from build123d import *

# Parameters (mm, degrees)
F1_DEPTH = 35
F2_DEPTH = 22.5
F5_DEPTH = 2
F7_D     = 2.4
F7_DEPTH = 18
F7_TIP   = 0.7210327428
F10_D    = 5


with BuildPart() as f1:
    # F0 (on Front) → F1 (new body, symmetric)
    with BuildSketch(Plane.XZ):
        with BuildLine():
            ThreePointArc((-74.9516211859, 11.7238655704), (-51.6668855763, 17.075104802), (-41.558504512, -4.5728813857))
            Line((-41.558504512, -4.5728813857), (-28.4346174449, -4.5728813857))
            Line((-28.4346174449, -4.5728813857), (-28.4346174449, -17.4488071352))
            Line((-28.4346174449, -17.4488071352), (-26.8566174449, -19.9622381479))
            Line((-26.8566174449, -19.9622381479), (-13.633294031, -19.9622381479))
            Line((-13.633294031, -19.9622381479), (-12.0557677819, -17.4488071352))
            Line((-12.0557677819, -17.4488071352), (-12.0557677819, -3.6602381479))
            Line((-12.0557677819, -3.6602381479), (8.6728588212, -3.6602381479))
            Line((8.6728588212, -3.6602381479), (8.6728588212, 8.3482577465))
            Line((8.6728588212, 8.3482577465), (22.1839677542, 8.3482577465))
            Line((22.1839677542, 8.3482577465), (22.1839677542, -4.337257977))
            Line((22.1839677542, -4.337257977), (41.558504512, -4.5728813857))
            Line((41.558504512, -4.5728813857), (44.6673956605, -4.5728813857))
            ThreePointArc((44.6673956605, -4.5728813857), (51.5748749774, 13.6021052912), (70.9240066517, 11.6904267961))
            Line((70.9240066517, 11.6904267961), (74.9777809213, 11.6904267961))
            Line((74.9777809213, 11.6904267961), (74.9516211859, 16.0203691918))
            Line((74.9516211859, 16.0203691918), (65.3270802818, 20.3168728132))
            Line((65.3270802818, 20.3168728132), (-65.3270802818, 20.3168728132))
            Line((-65.3270802818, 20.3168728132), (-74.9516211859, 16.0203691918))
            Line((-74.9516211859, 16.0203691918), (-74.9516211859, 11.7238655704))
        make_face()
    extrude(amount=F1_DEPTH, both=True)

    # F0 (on Front) → F2 (join, symmetric)
    with BuildSketch(Plane.XZ):
        with BuildLine():
            ThreePointArc((-68, -13.8564064606), (-75.8989864476, -1.7950570853), (-70.888111686, 11.7238655704))
            Line((-70.888111686, 11.7238655704), (-74.9516211859, 11.7238655704))
            ThreePointArc((-74.9516211859, 11.7238655704), (-78.6540953163, -3.6089787931), (-69.5, -16.4544826719))
            Line((-69.5, -16.4544826719), (-68, -13.8564064606))
        make_face()
        with BuildLine():
            ThreePointArc((-44.6673956605, -4.5728813857), (-47.4441819952, -9.9172291609), (-52, -13.8564064606))
            Line((-52, -13.8564064606), (-50.5, -16.4544826719))
            ThreePointArc((-50.5, -16.4544826719), (-44.818600038, -11.4247579927), (-41.558504512, -4.5728813857))
            Line((-41.558504512, -4.5728813857), (-44.6673956605, -4.5728813857))
        make_face()
        with BuildLine():
            ThreePointArc((-70.888111686, 11.7238655704), (-51.5540323778, 13.5891732981), (-44.6673956605, -4.5728813857))
            Line((-44.6673956605, -4.5728813857), (-41.558504512, -4.5728813857))
            ThreePointArc((-41.558504512, -4.5728813857), (-51.6668855763, 17.075104802), (-74.9516211859, 11.7238655704))
            Line((-74.9516211859, 11.7238655704), (-70.888111686, 11.7238655704))
        make_face()
        with BuildLine():
            ThreePointArc((52, -13.8564064606), (47.4441819952, -9.9172291609), (44.6673956605, -4.5728813857))
            Line((44.6673956605, -4.5728813857), (41.558504512, -4.5728813857))
            ThreePointArc((41.558504512, -4.5728813857), (44.818600038, -11.4247579927), (50.5, -16.4544826719))
            Line((50.5, -16.4544826719), (52, -13.8564064606))
        make_face()
        with BuildLine():
            ThreePointArc((69.5, -16.4544826719), (78.6500515267, -3.629817909), (74.9777809213, 11.6904267961))
            Line((74.9777809213, 11.6904267961), (70.9240066517, 11.6904267961))
            ThreePointArc((70.9240066517, 11.6904267961), (75.8962158798, -1.8194286745), (68, -13.8564064606))
            Line((68, -13.8564064606), (69.5, -16.4544826719))
        make_face()
    extrude(amount=F2_DEPTH, both=True)

    # F4 (on offset) → F5 (join)
    with BuildSketch(Plane.XZ.offset(22.5)):
        with BuildLine():
            ThreePointArc((-66.2250077663, -10.764406164), (-60.0242756476, 12.4257611455), (-53.8000638867, -10.7581152906))
            Line((-53.8000638867, -10.7581152906), (-50.5566579219, -16.7363728506))
            ThreePointArc((-50.5566579219, -16.7363728506), (-59.9985634557, 19.2255688342), (-69.5131042914, -16.7172238027))
            Line((-69.5131042914, -16.7172238027), (-66.2250077663, -10.764406164))
        make_face()
        with BuildLine():
            ThreePointArc((69.5131042914, -16.7172238027), (59.9985634557, 19.2255688342), (50.5566579219, -16.7363728506))
            Line((50.5566579219, -16.7363728506), (53.8000638867, -10.7581152906))
            ThreePointArc((53.8000638867, -10.7581152906), (60.0242756476, 12.4257611455), (66.2250077663, -10.764406164))
            Line((66.2250077663, -10.764406164), (69.5131042914, -16.7172238027))
        make_face()
    extrude(amount=F5_DEPTH)

    # F7 (one way)
    with BuildSketch(Plane.YZ.offset(-12.0557677819)):
        with Locations((-20, -11.9100315496), (20, -11.9100315496)):
            Circle(F7_D / 2)
    extrude(amount=-F7_DEPTH, mode=Mode.SUBTRACT)
    with Locations(Plane.YZ.offset(-12.0557677819)):
        with Locations((-20, -11.9100315496), (20, -11.9100315496)):
            with Locations((0, 0, -(F7_DEPTH + F7_TIP / 2))):  # 118° drill point
                Cone(0, F7_D / 2, F7_TIP, mode=Mode.SUBTRACT)

    # F10 (through all)
    with Locations(Plane.XY.offset(20.3168728132)):
        with Locations((0, 0)):
            Hole(F10_D / 2)


solid = f1.part
Here's how the part is built. I have some questions about the finished solid (model axes, mm). A direction names the side the tool comes from. Give positions to 0.01 mm unless a question says otherwise; leave off trailing zeros. Loops run counter-clockwise (first coordinate to the right, second up) from the corner with the lowest first, then second, coordinate; pieces in that order, holes last. Notation, with made-up numbers: (-38, 29.25) -> (-20, 29.25) arc R11 cw to (-20, 44.25) -> close; hole circle Ø4 at (5, 69.5). An arc over 180 degrees is marked (long way). Answer as a JSON object with one key per item and string values. Group by question number.
Item 1: Imagine slicing it at D-D on y = -12. Write out the boundary of the cut face in (x, z).
Item 2: I need wall thicknesses on L1, parallel to X at y = -23, z = 0; L2, parallel to X at y = 9, z = 0; L3, parallel to X at y = 2, z = 0. Which ranges of each line are inside material? Lowest first, please.
Item 3: Imagine slicing it at A-A on x = 0. Write out the boundary of the cut face in (y, z).
Item 4: Imagine slicing it at C-C on y = -28. Write out the boundary of the cut face in (x, z), then the cut area to 3 significant figures.
Item 5: Thinking about a two-plate mould opening in X: for faces 1 (the flat face through (73, 29, 11.69)), 2 (the cylindrical face through (-51.99, 28.66, 17.23)), 3 (the cylindrical face through (-78.952, -23.486, -3.335)), which applies, pulls with the +X half, pulls with the -X half, needs draft (parallel to the pull), parting line crosses it, or undercut?
Item 6: Will these pins go through, and if not, where does the flat tip stop? pin 1 (6.5 mm diameter, centred on x = -35, y = -15.5, fed in from -Z); pin 2 (16.5 mm diameter, centred on x = 2, y = -9, fed in from -Z); pin 3 (14 mm diameter, centred on y = -4, z = -12.5, fed in from -X).
Item 7: Imagine slicing it at B-B on z = 0. Give the number of separate pieces and of enclosed holes in the cut face, then the cut area to 3 significant figures.
Item 8: On a 3-axis mill with a long thin cutter (end or side, diameter ignored), from which of +Z, -Z, +X, -X, +Y, -Y can I reach the whole of each face in a straight line? I mean faces 4 (the flat face through (73, -30, 11.69)), 5 (the flat face through (-28.435, 0, -11)), 6 (the flat face through (43, 29, -4.573)). Say none if no direction works.
Answer list:
{
 "1": {"outline": "(-74.95, 11.72) arc R19 ccw to (-69.5, -16.45) -> (-68, -13.86) arc R16 cw (long way) to (-52, -13.86) -> (-50.5, -16.45) arc R19 ccw to (-41.56, -4.57) -> (-28.43, -4.57) -> (-28.43, -17.45) -> (-26.86, -19.96) -> (-13.63, -19.96) -> (-12.06, -17.45) -> (-12.06, -3.66) -> (8.67, -3.66) -> (8.67, 8.35) -> (22.18, 8.35) -> (22.18, -4.34) -> (41.56, -4.57) arc R19 ccw to (50.5, -16.45) -> (52, -13.86) arc R16 cw (long way) to (68, -13.86) -> (69.5, -16.45) arc R19 ccw to (74.98, 11.69) -> (74.95, 16.02) -> (65.33, 20.32) -> (-65.33, 20.32) -> (-74.95, 16.02) -> close"},
 "2": {"L1": "x = -79.24 to -72.44, -47.59 to 8.67, 22.18 to 47.59, 72.44 to 79.24", "L2": "x = -79 to -76, -44 to 8.67, 22.18 to 44, 76 to 79", "L3": "x = -79 to -76, -44 to -1.5, 1.5 to 8.67, 22.18 to 44, 76 to 79"},
 "3": {"outline": "(-35, -3.66) -> (-2.5, -3.66) -> (-2.5, 20.32) -> (-35, 20.32) -> close; (2.5, -3.66) -> (35, -3.66) -> (35, 20.32) -> (2.5, 20.32) -> close"},
 "4": {"outline": "(-74.95, 11.72) arc R19 cw to (-41.56, -4.57) -> (-28.43, -4.57) -> (-28.43, -17.45) -> (-26.86, -19.96) -> (-13.63, -19.96) -> (-12.06, -17.45) -> (-12.06, -3.66) -> (8.67, -3.66) -> (8.67, 8.35) -> (22.18, 8.35) -> (22.18, -4.34) -> (41.56, -4.57) -> (44.67, -4.57) arc R16 cw to (70.92, 11.69) -> (74.98, 11.69) -> (74.95, 16.02) -> (65.33, 20.32) -> (-65.33, 20.32) -> (-74.95, 16.02) -> close", "area": "2,500 mm2"},
 "5": {"face 1": "needs draft", "face 2": "undercut", "face 3": "pulls with the -X half"},
 "6": {"pin 1": "stops at z = -4.57", "pin 2": "stops at z = -3.66", "pin 3": "stops at x = -78.19"},
 "7": {"separate pieces": "4", "enclosed holes": "1", "area": "5,440 mm2"},
 "8": {"face 4": "-Z, +X, -Y", "face 5": "-Z, +Y, -Y", "face 6": "-Z, +X, +Y"}
}
